```python
from build123d import *

# Parameters (mm, degrees)
SKETCH1_W           = 1.2
SKETCH1_H           = 0.75
SKETCH1_W_2         = 4.2
SKETCH1_W_3         = 8
SKETCH1_H_2         = 2.733563445
SKETCH2_W           = 9.36396103
SKETCH2_H           = 9.36396103
SKETCH2_R           = 1
BOSS_EXTRUDE1_DEPTH = 2
FILLET1_R           = 1.5
SKETCH3_R           = 1
CUT_EXTRUDE1_DEPTH  = 2


with BuildPart() as part:
    # Sketch1 → Revolve1 (revolve)
    with BuildSketch(Plane(origin=(0, 0, 0), x_dir=(0, 0, -1), z_dir=(1, 0, 0))):
        with Locations((-0.6, 0.375)):
            Rectangle(SKETCH1_W, SKETCH1_H)
        with Locations((2.1, 0.375)):
            Rectangle(SKETCH1_W_2, SKETCH1_H)
        with Locations((8.2, 0.375)):
            Rectangle(SKETCH1_W_3, SKETCH1_H)
        with Locations((14.3, 0.375)):
            Rectangle(SKETCH1_W_2, SKETCH1_H)
        Polygon((4.2, 3.483563445), (4.2, 0.75), (12.2, 0.75), (12.2, 8.9), (4.2, 8.9), align=None)
        with Locations((2.1, 2.116781722)):
            Rectangle(SKETCH1_W_2, SKETCH1_H_2)
    revolve(axis=Axis((0, 0, 1.2), (0, 0, -1)))

    # Sketch2 → Boss-Extrude1 (add)
    with BuildSketch(Plane.XY):
        Rectangle(SKETCH2_W, SKETCH2_H)
        with Locations((3.181980515, 3.181980515)):
            Circle(SKETCH2_R, mode=Mode.SUBTRACT)
        with Locations((3.181980515, -3.181980515)):
            Circle(SKETCH2_R, mode=Mode.SUBTRACT)
        with Locations((-3.181980515, -3.181980515)):
            Circle(SKETCH2_R, mode=Mode.SUBTRACT)
        with Locations((-3.181980515, 3.181980515)):
            Circle(SKETCH2_R, mode=Mode.SUBTRACT)
    extrude(amount=-BOSS_EXTRUDE1_DEPTH)

    # Fillet1
    fillet1_edges = [part.edges().sort_by_distance(p)[0] for p in [
        (4.681980515, 4.681980515, -1),
        (4.681980515, -4.681980515, -1),
        (-4.681980515, -4.681980515, -1),
        (-4.681980515, 4.681980515, -1),
    ]]
    fillet(fillet1_edges, radius=FILLET1_R)

    # Sketch3 → Cut-Extrude1 (cut)
    with BuildSketch(Plane(origin=(0, 0, -12.2), x_dir=(-1, 0, 0), z_dir=(0, 0, -1))):
        with Locations((0, 2.5)):
            Circle(SKETCH3_R)
        with Locations((2.5, 0)):
            Circle(SKETCH3_R)
        with Locations((0, -2.5)):
            Circle(SKETCH3_R)
        with Locations((-2.5, 0)):
            Circle(SKETCH3_R)
    extrude(amount=-CUT_EXTRUDE1_DEPTH, mode=Mode.SUBTRACT)


solid = part.part
```
For this review, take the finished solid that the model builds, in its own axes (mm). A direction names the side the tool comes from. Round coordinates to 2 decimals unless told otherwise and drop trailing zeros. Write each loop counter-clockwise with the first axis right and the second up, starting at its lowest first coordinate (ties: lowest second). Pieces come first, ordered by that corner, then holes. Notation, with made-up numbers: (-35, 67) -> (-7, 67) arc R31 cw to (-7, 93) -> close; hole circle Ø1 at (75, 31). An arc over 180 degrees is marked (long way). One line per question, with ' | ' between items. Start each with the question number.
(1) For line 1 along Z through (x, y) = (4.5, 0.25); line 2 along Z through (x, y) = (-3, 7.25); line 3 along Y through (x, z) = (2.5, -11.75), list the stretches that pass through material, from the lowest coordinate up. Write a range as from..to.
(2) Mouldability with a two-part tool opening along Y and no side actions: class faces 1 (the face through (4.231, -4.254, -1.014)), 2 (the face through (0.217, -3.476, -11.214)), 3 (the face through (0, 0, 1.2)), 4 (the face through (0, 3, -10.2)) as released by +Y, released by -Y, zero draft, split by the parting line, or undercut.
(3) Add section C-C, the plane y = 0. Write out the cut boundary in (x, z).
(4) Insertion check: P1, Ø3, axis at x = -3.18, y = 3.18, coming from the -Z side; P2, Ø5.5, axis at x = 2, y = 2, coming from the +Z side; P3, Ø4, axis at y = 0, z = -14.5, coming from the +X side; P4, Ø4, axis at y = 6, z = -4, coming from the +X side. Each pin has a flat end and moves straight along its axis. Give the tip position at first contact, or say it passes through.
(5) Tool access review of faces 5 (the face through (-4.682, 0, -1)), 6 (the face through (4.682, 0, -1)), 7 (the face through (-2.258, -3.565, -0.986)), 8 (the face through (3, 0, -10.2)), 9 (the face through (0, -4.682, -1)): name each direction out of +Z, -Z, +X, -X, +Y, -Y from which nothing blocks a thin tool from reaching the whole face with its end or side.
(6) Add section A-A, the plane y = 2.5. Give the number of separate pieces and of enclosed holes in the cut face, plus the area to 3 significant figures.
Answer list:
1) line 1: -12.2..-4.2, -2..0 | line 2: -12.2..-4.2 | line 3: -8.54..-1, 1..8.54
2) face 1: released by -Y | face 2: undercut | face 3: zero draft | face 4: undercut
3) outline: (-8.9, -12.2) -> (-3.5, -12.2) -> (-3.5, -10.2) -> (-1.5, -10.2) -> (-1.5, -12.2) -> (-0.75, -12.2) -> (-0.75, -16.4) -> (0.75, -16.4) -> (0.75, -12.2) -> (1.5, -12.2) -> (1.5, -10.2) -> (3.5, -10.2) -> (3.5, -12.2) -> (8.9, -12.2) -> (8.9, -4.2) -> (3.48, -4.2) -> (3.48, -2) -> (4.68, -2) -> (4.68, 0) -> (0.75, 0) -> (0.75, 1.2) -> (-0.75, 1.2) -> (-0.75, 0) -> (-4.68, 0) -> (-4.68, -2) -> (-3.48, -2) -> (-3.48, -4.2) -> (-8.9, -4.2) -> close
4) P1: z = -12.2 | P2: z = 1.2 | P3: x = 0.75 | P4: x = 7.95
5) face 5: +Z, -X, +Y, -Y | face 6: +Z, +X, +Y, -Y | face 7: +Z | face 8: -Z | face 9: +Z, +X, -X, -Y
6) separate pieces: 3 | enclosed holes: 0 | area: 156 mm²
